Can you work these out from the model? Positions are in its coordinate system, mm. Face numbers are marked on the shaded views. A direction names the side the tool comes from. Give positions to 0.01 mm unless a question says otherwise; leave off trailing zeros. Write each loop counter-clockwise with the first axis right and the second up, starting at its lowest first coordinate (ties: lowest second). Pieces come first, ordered by that corner, then holes.
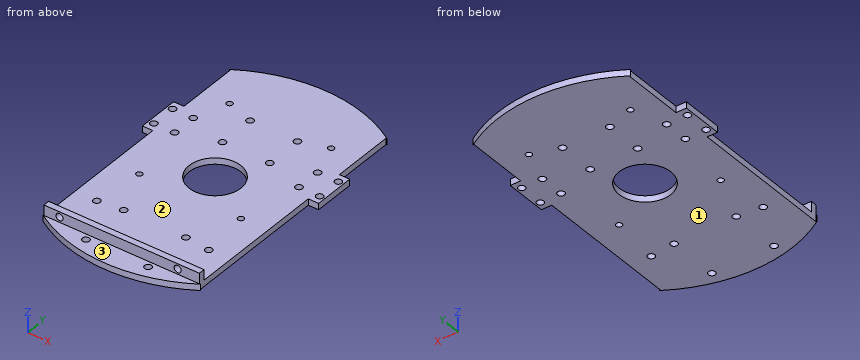
from build123d import *

# Parameters (mm, degrees)
SKETCH_R        = 71
PAD_DEPTH       = 3
SKETCH001_W     = 52.5
SKETCH001_H     = 120
POCKET_DEPTH    = 3.001
SKETCH002_W     = 55.43
SKETCH002_H     = 120
POCKET001_DEPTH = 3.001
SKETCH003_R     = 12.5
POCKET002_DEPTH = 3.001
SKETCH004_R     = 1.7
HOLE_DEPTH      = 3.001
SKETCH005_W     = 15
SKETCH005_H     = 20
PAD001_DEPTH    = 3
SKETCH006_W     = 15
SKETCH006_H     = 20
PAD002_DEPTH    = 3
SKETCH007_W     = 75
SKETCH007_H     = 3
PAD003_DEPTH    = 8
SKETCH008_R     = 1.7
HOLE001_DEPTH   = 8.001
SKETCH010_R     = 1.45
HOLE002_DEPTH   = 8.001
SKETCH011_R     = 1.7
HOLE003_DEPTH   = 8.001
SKETCH013_R     = 1.7
HOLE004_DEPTH   = 8.001
SKETCH014_R     = 1.7
HOLE005_DEPTH   = 71.001


with BuildPart() as part:
    # Sketch → Pad (new body)
    with BuildSketch(Plane.XY):
        Circle(SKETCH_R)
    extrude(amount=PAD_DEPTH)

    # Sketch001 → Pocket (cut, through all)
    with BuildSketch(Plane.XY):
        with Locations((63.75, 0)):
            Rectangle(SKETCH001_W, SKETCH001_H)
    extrude(amount=POCKET_DEPTH, mode=Mode.SUBTRACT)

    # Sketch002 → Pocket001 (cut, through all)
    with BuildSketch(Plane.XY):
        with Locations((-65.215, 0)):
            Rectangle(SKETCH002_W, SKETCH002_H)
    extrude(amount=POCKET001_DEPTH, mode=Mode.SUBTRACT)

    # Sketch003 → Pocket002 (cut, through all)
    with BuildSketch(Plane.XY):
        Circle(SKETCH003_R)
    extrude(amount=POCKET002_DEPTH, mode=Mode.SUBTRACT)

    # Sketch004 → Hole (cut, through all)
    with BuildSketch(Plane.XY):
        with Locations((-15, -38.7)):
            Circle(SKETCH004_R)
        with Locations((15, -38.7)):
            Circle(SKETCH004_R)
        with Locations((-15, -63)):
            Circle(SKETCH004_R)
        with Locations((15, -63)):
            Circle(SKETCH004_R)
    extrude(amount=HOLE_DEPTH, mode=Mode.SUBTRACT)

    # Sketch005 → Pad001 (join)
    with BuildSketch(Plane.XY):
        with Locations((35, 20)):
            Rectangle(SKETCH005_W, SKETCH005_H)
    extrude(amount=PAD001_DEPTH)

    # Sketch006 → Pad002 (join)
    with BuildSketch(Plane.XY):
        with Locations((-35, 20)):
            Rectangle(SKETCH006_W, SKETCH006_H)
    extrude(amount=PAD002_DEPTH)

    # Sketch007 → Pad003 (join)
    with BuildSketch(Plane.XY):
        with Locations((0, -58.5)):
            Rectangle(SKETCH007_W, SKETCH007_H)
    extrude(amount=PAD003_DEPTH)

    # Sketch008 → Hole001 (cut, through all)
    with BuildSketch(Plane.XY):
        with Locations((-27, -40)):
            Circle(SKETCH008_R)
        with Locations((27, -40)):
            Circle(SKETCH008_R)
    extrude(amount=HOLE001_DEPTH, mode=Mode.SUBTRACT)

    # Sketch010 → Hole002 (cut, through all)
    with BuildSketch(Plane.XY):
        with Locations((-24.5, -16)):
            Circle(SKETCH010_R)
        with Locations((24.5, -16)):
            Circle(SKETCH010_R)
        with Locations((24.5, 42)):
            Circle(SKETCH010_R)
        with Locations((-24.5, 42)):
            Circle(SKETCH010_R)
    extrude(amount=HOLE002_DEPTH, mode=Mode.SUBTRACT)

    # Sketch011 → Hole003 (cut, through all)
    with BuildSketch(Plane.XY):
        with Locations((-30, 26)):
            Circle(SKETCH011_R)
        with Locations((-40, 26)):
            Circle(SKETCH011_R)
        with Locations((-30, 14)):
            Circle(SKETCH011_R)
        with Locations((-40, 14)):
            Circle(SKETCH011_R)
        with Locations((30, 26)):
            Circle(SKETCH011_R)
        with Locations((40, 26)):
            Circle(SKETCH011_R)
        with Locations((30, 14)):
            Circle(SKETCH011_R)
        with Locations((40, 14)):
            Circle(SKETCH011_R)
    extrude(amount=HOLE003_DEPTH, mode=Mode.SUBTRACT)

    # Sketch013 → Hole004 (cut, through all)
    with BuildSketch(Plane.XY):
        with Locations((-11.43, 37.78)):
            Circle(SKETCH013_R)
        with Locations((11.43, 37.78)):
            Circle(SKETCH013_R)
        with Locations((-11.43, 20)):
            Circle(SKETCH013_R)
        with Locations((11.43, 20)):
            Circle(SKETCH013_R)
    extrude(amount=HOLE004_DEPTH, mode=Mode.SUBTRACT)

    # Sketch014 → Hole005 (cut, through all)
    with BuildSketch(Plane.XZ):
        with Locations((-30, 5.5)):
            Circle(SKETCH014_R)
        with Locations((27, 5.5)):
            Circle(SKETCH014_R)
    extrude(amount=HOLE005_DEPTH, mode=Mode.SUBTRACT)


solid = part.part
(1) Imagine slicing it at D-D, the plane z = 1.25. Give the number of separate pieces and of enclosed holes in the cut face, plus the area to 3 significant figures.
Returned:
separate pieces: 1
enclosed holes: 23
area: 9,650 mm2
(2) Will these pins go through, and if not, where does the flat tip stop? P1, Ø5.5, axis at x = 40, y = 14, coming from the +Z side; P2, Ø12, axis at x = 15, y = 33.5, coming from the -Z side; P3, Ø3.5, axis at x = 40, z = 1.5, coming from the -Y side; P4, Ø1.5, axis at y = 51.5, z = 1, coming from the -X side.
Returned:
P1: stops at z = 3
P2: stops at z = 0
P3: stops at y = 10
P4: stops at x = -37.5
(3) Imagine slicing it at B-B, the plane y = 0. Write out the boundary of the cut face in (x, z).
Returned:
outline: (-37.5, 0) - (-12.5, 0) - (-12.5, 3) - (-37.5, 3) - close; (12.5, 0) - (37.5, 0) - (37.5, 3) - (12.5, 3) - close
(4) For the marked faces 1, 2 and 3, which set-ups out of +Z, -Z, +X, -X, +Y, -Y let a thin tool reach every point of the face, with its end or its side?
Returned:
face 1: -Z, +X, -X, +Y, -Y
face 2: +Z, +X, -X, +Y
face 3: +Z, +X, -X, -Y
(5) Imagine slicing it at C-C, the plane x = -40. Write out the boundary of the cut face in (y, z), plus the area to 3 significant figures.
Returned:
outline: (10, 0) - (12.3, 0) - (12.3, 3) - (10, 3) - close; (15.7, 0) - (24.3, 0) - (24.3, 3) - (15.7, 3) - close; (27.7, 0) - (30, 0) - (30, 3) - (27.7, 3) - close
area: 39.6 mm2
(6) Imagine slicing it at A-A, the plane y = 37.78. Write out the boundary of the cut face in (x, z).
Returned:
outline: (-37.5, 0) - (-13.13, 0) - (-13.13, 3) - (-37.5, 3) - close; (-9.73, 0) - (9.73, 0) - (9.73, 3) - (-9.73, 3) - close; (13.13, 0) - (37.5, 0) - (37.5, 3) - (13.13, 3) - close
(7) If I drill on L1, parallel to X at y = -58, z = 5.5; L2, parallel to Y at x = 40, z = 1.1; L3, parallel to X at y = -16, z = 1.4, over which ranges is the centre line in solid material (lowest first)?
Returned:
L1: x = -37.5 to -31.7, -28.3 to 25.3, 28.7 to 37.5
L2: y = 10 to 12.3, 15.7 to 24.3, 27.7 to 30
L3: x = -37.5 to -25.95, -23.05 to 23.05, 25.95 to 37.5
